Verification items for the finished model (mm, model axes). A direction names the side the tool comes from. Round coordinates to 2 decimals unless told otherwise and drop trailing zeros. Write each loop counter-clockwise with the first axis right and the second up, starting at its lowest first coordinate (ties: lowest second). Pieces come first, ordered by that corner, then holes. Notation, with made-up numbers: (54.25, 8.25) - (85.25, 8.25) arc R22 ccw to (85.25, 43.25) - close; hole circle Ø6 at (40, 22). An arc over 180 degrees is marked (long way). Answer as a JSON object with one key per item and string values. Group by question number.
1) Section check D-D (y = 34.5). Enter the section's corners in (x, z).
2) Mould release check, pull along Z, two halves, no side actions. Record for faces 1 (the cylindrical face through (23.586, 0.021, 25.792)), 2 (the flat face through (-6, 11, 55)), 3 (the flat face through (-25, 0, 27)): +Z half, -Z half, draft (parallel to the pull), parting line (faces both ways), or undercut.
3) Section check C-C (z = 36.5). Enter the section's corners in (x, y), then the cut area to 3 significant figures.
4) Section check B-B (x = 0). Enter the section's corners in (y, z), then the cut area to 3 significant figures.
5) Go/stop test with flat-tipped pins: pin 1 Ø6.5 at (x, z) = (-19.5, 14) entering from +Y; pin 2 Ø5 at (x, z) = (22, 26) entering from +Y; pin 3 Ø18.5 at (x, y) = (5, 17.5) entering from -Z; pin 4 Ø1.9 at (x, y) = (-13.42, 31.25) entering from +Z. Record where each tip stops, or that it passes through.
6) Section check A-A (z = 26). Enter the section's corners in (x, y), then the cut area to 3 significant figures.
7) Set-up check for faces 4 (the cylindrical face through (-14.223, 6.355, 27.885)), 5 (the flat face through (10, 14, 50)), 6 (the cylindrical face through (-20.414, 0.021, 38.792)), 7 (the cylindrical face through (14.2, 6.3, 27.9)): record each of +Z, -Z, +X, -X, +Y, -Y from which the full face is reachable in a straight line by a thin tool's end or side.
8) Thickness scan on line 1 (X direction, y = -0.15, z = 39); line 2 (Y direction, x = 0, z = 12.5); line 3 (Y direction, x = 16, z = 19). Record the ranges inside material, lowest first.
```python
from build123d import *

# Parameters (mm, degrees)
IZIM1_R                     = 18.65
IZIM1_W                     = 50
IZIM1_H                     = 3
Y_KSEKLIK_EKSTR_ZYON4_DEPTH = 55
RADYUS1_R                   = 3
RADYUS2_R                   = 3
IZIM7_R                     = 1.6
KES_EKSTR_ZYON1_DEPTH       = 55
IZIM8_R                     = 1.6
KES_EKSTR_ZYON2_DEPTH       = 55
Y_KSEKLIK_EKSTR_ZYON5_START = -5
IZIM10_R                    = 18.65
IZIM10_R_2                  = 13.5
IZIM10_R_3                  = 1.6
Y_KSEKLIK_EKSTR_ZYON5_DEPTH = 5


with BuildPart() as part:
    # Çizim1 → Yükseklik-Ekstrüzyon4 (new body)
    # profile 1 of 4: a face of its own
    with BuildSketch(Plane.XY):
        with BuildLine():
            ThreePointArc((-10.528747961, 42.81697353), (-21.902220366, 25.57189359), (-13.964240044, 6.5))
            ThreePointArc((-13.964240044, 6.5), (-7.416198487, 2.787684823), (0, 1.5))
            ThreePointArc((0, 1.5), (7.416198487, 2.787684823), (13.964240044, 6.5))
            ThreePointArc((13.964240044, 6.5), (19.889862757, 14.098225725), (22, 23.5))
            ThreePointArc((22, 23.5), (18.916030968, 34.733155052), (10.528747961, 42.81697353))
            Line((10.528747961, 42.81697353), (-10.528747961, 42.81697353))
        make_face()
        with Locations((0, 23.5)):
            Circle(IZIM1_R, mode=Mode.SUBTRACT)
    # profile 2 of 4: a face of its own
    with BuildSketch(Plane.XY):
        Rectangle(IZIM1_W, IZIM1_H)
    # profile 3 of 4: a face of its own
    with BuildSketch(Plane.XY):
        with BuildLine():
            ThreePointArc((0, 1.5), (-7.416198487, 2.787684823), (-13.964240044, 6.5))
            Line((-13.964240044, 6.5), (-13.964240044, 1.5))
            Line((-13.964240044, 1.5), (0, 1.5))
        make_face()
    # profile 4 of 4: a face of its own
    with BuildSketch(Plane.XY):
        with BuildLine():
            ThreePointArc((13.964240044, 6.5), (7.416198487, 2.787684823), (0, 1.5))
            Line((0, 1.5), (13.964240044, 1.5))
            Line((13.964240044, 1.5), (13.964240044, 6.5))
        make_face()
    extrude(amount=Y_KSEKLIK_EKSTR_ZYON4_DEPTH)

    # Radyus1
    radyus1_edges = [part.edges().sort_by_distance(p)[0] for p in [
        (13.964240044, 6.5, 27.5),
        (13.964240044, 1.5, 27.5),
    ]]
    fillet(radyus1_edges, radius=RADYUS1_R)

    # Radyus2
    radyus2_edges = [part.edges().sort_by_distance(p)[0] for p in [
        (-13.964240044, 1.5, 27.5),
        (-13.964240044, 6.5, 27.5),
    ]]
    fillet(radyus2_edges, radius=RADYUS2_R)

    # Çizim7 → Kes-Ekstrüzyon1 (cut)
    with BuildSketch(Plane(origin=(0, 1.5, 0), x_dir=(1, 0, 0), z_dir=(0, 1, 0))):
        with Locations(Location((-22, -13, 0), (0, 0, 270))):
            Circle(IZIM7_R)
        with Locations(Location((-22, -26, 0), (0, 0, 270))):
            Circle(IZIM7_R)
        with Locations(Location((-22, -39, 0), (0, 0, 270))):
            Circle(IZIM7_R)
    extrude(amount=-KES_EKSTR_ZYON1_DEPTH, mode=Mode.SUBTRACT)

    # Çizim8 → Kes-Ekstrüzyon2 (cut)
    with BuildSketch(Plane(origin=(0, 1.5, 0), x_dir=(1, 0, 0), z_dir=(0, 1, 0))):
        with Locations(Location((22, -13, 0), (0, 0, 270))):
            Circle(IZIM8_R)
        with Locations(Location((22, -26, 0), (0, 0, 270))):
            Circle(IZIM8_R)
        with Locations(Location((22, -39, 0), (0, 0, 270))):
            Circle(IZIM8_R)
    extrude(amount=-KES_EKSTR_ZYON2_DEPTH, mode=Mode.SUBTRACT)

    # Çizim10 → Yükseklik-Ekstrüzyon5 (add)
    with BuildSketch(Plane.XY.offset(55).offset(Y_KSEKLIK_EKSTR_ZYON5_START)):
        with Locations((0, 23.5)):
            Circle(IZIM10_R)
        with Locations((0, 23.5)):
            Circle(IZIM10_R_2, mode=Mode.SUBTRACT)
        with Locations((-13.42, 31.25)):
            Circle(IZIM10_R_3, mode=Mode.SUBTRACT)
        with Locations((-13.42, 15.75)):
            Circle(IZIM10_R_3, mode=Mode.SUBTRACT)
        with Locations((13.42, 31.25)):
            Circle(IZIM10_R_3, mode=Mode.SUBTRACT)
        with Locations((13.42, 15.75)):
            Circle(IZIM10_R_3, mode=Mode.SUBTRACT)
    extrude(amount=Y_KSEKLIK_EKSTR_ZYON5_DEPTH)


solid = part.part
```
Returned:
{
 "1": {"outline": "(-19.05, 0) - (-15.06, 0) - (-15.06, 50) - (-7.83, 50) - (-7.83, 55) - (-19.05, 55) - close; (7.83, 50) - (15.06, 50) - (15.06, 0) - (19.05, 0) - (19.05, 55) - (7.83, 55) - close"},
 "2": {"face 1": "undercut", "face 2": "+Z half", "face 3": "draft"},
 "3": {"outline": "(-25, -1.5) - (25, -1.5) - (25, 1.5) - (16.96, 1.5) arc R3 cw to (13.96, 4.5) - (13.96, 5.14) arc R3 cw to (14.93, 7.34) arc R22 ccw to (10.53, 42.82) - (-10.53, 42.82) arc R22 ccw to (-14.93, 7.34) arc R3 cw to (-13.96, 5.14) - (-13.96, 4.5) arc R3 cw to (-16.96, 1.5) - (-25, 1.5) - close; hole circle Ø37.3 at (0, 23.5)", "area": "588 mm2"},
 "4": {"outline": "(-1.5, 0) - (4.85, 0) - (4.85, 50) - (10, 50) - (10, 55) - (-1.5, 55) - close; (37, 50) - (42.15, 50) - (42.15, 0) - (42.82, 0) - (42.82, 55) - (37, 55) - close", "area": "437 mm2"},
 "5": {"pin 1": "y = 38.33", "pin 2": "y = 33.69", "pin 3": "z = 50", "pin 4": "through"},
 "6": {"outline": "(-25, -1.5) - (-23.6, -1.5) - (-23.6, 1.5) - (-25, 1.5) - close; (-20.4, -1.5) - (20.4, -1.5) - (20.4, 1.5) - (16.96, 1.5) arc R3 cw to (13.96, 4.5) - (13.96, 5.14) arc R3 cw to (14.93, 7.34) arc R22 ccw to (10.53, 42.82) - (-10.53, 42.82) arc R22 ccw to (-14.93, 7.34) arc R3 cw to (-13.96, 5.14) - (-13.96, 4.5) arc R3 cw to (-16.96, 1.5) - (-20.4, 1.5) - close; (23.6, -1.5) - (25, -1.5) - (25, 1.5) - (23.6, 1.5) - close; hole circle Ø37.3 at (0, 23.5)", "area": "569 mm2"},
 "7": {"face 4": "+Z, -Z, -X", "face 5": "-Z", "face 6": "-Y", "face 7": "+Z, -Z, +X"},
 "8": {"line 1": "-25 to -23.6, -20.4 to 20.4, 23.6 to 25", "line 2": "-1.5 to 4.85, 42.15 to 42.82", "line 3": "-1.5 to 1.66, 8.4 to 13.92, 33.08 to 38.6"}
}
